```python
from build123d import *

# Parameters (mm, degrees)
EXTRUDE_1_DEPTH     = 4.95
SKETCH_2_R          = 0.5
CUT_EXTRUDE_1_DEPTH = 0.5
CUT_EXTRUDE_2_REACH = 16.197
CUT_EXTRUDE_3_REACH = 16.197
SKETCH_5_R          = 2.8
SKETCH_5_R_2        = 0.4
EXTRUDE_2_DEPTH     = 1.42
CHAMFER_1_SIZE      = 0.5
CHAMFER_1_SIZE2     = 0.466257543


with BuildPart() as part:
    # Эскиз1 → Бобышка-Вытянуть1 (new, symmetric)
    with BuildSketch(Plane(origin=(0, 0, 0), x_dir=(0, 0, -1), z_dir=(1, 0, 0))):
        Polygon((0, 1.59), (-4.55, 1.59), (-4.55, 0.59), (-4.55, 0.34), (-4.55, -1.59), (0, -1.59), align=None)
        Polygon((4.55, 1.59), (0, 1.59), (0, -1.59), (4.55, -1.59), (4.55, 0.34), (4.55, 0.59), align=None)
        Polygon((-4.55, 0.34), (-4.55, 0.59), (-6.25, 0.59), (-6.25, -4.56), (-6, -4.56), (-6, 0.34), align=None)
        Polygon((6.25, 0.59), (4.55, 0.59), (4.55, 0.34), (6, 0.34), (6, -4.56), (6.25, -4.56), align=None)
    extrude(amount=EXTRUDE_1_DEPTH, both=True)

    # Эскиз2 → Вырез-Вытянуть1 (cut)
    with BuildSketch(Plane(origin=(0, 1.59, 0), x_dir=(1, 0, 0), z_dir=(0, 1, 0))):
        with Locations(Location((-4, -3.55, 0), (0, 0, 270))):
            Circle(SKETCH_2_R)
    extrude(amount=-CUT_EXTRUDE_1_DEPTH, mode=Mode.SUBTRACT)

    # Вырез-Вытянуть2: up to this face of the body (flat: up to its plane)
    cut_extrude_2_end = Plane(part.part.faces().sort_by_distance((0, -0.625, 4.55))[0])
    # Эскиз3 → Вырез-Вытянуть2 (cut, up to the picked face)
    with BuildSketch(Plane.XY.offset(6.25), mode=Mode.PRIVATE) as cut_extrude_2_sk1:
        Polygon((-3, -1.59), (-3, 0.59), (-4.95, 0.59), (-4.95, -4.56), (-2.73, -4.56), (-2.73, -1.59), align=None)
    cut_extrude_2_tool1 = split(extrude(cut_extrude_2_sk1.sketch, amount=-CUT_EXTRUDE_2_REACH, mode=Mode.PRIVATE), bisect_by=cut_extrude_2_end, keep=Keep.BOTH, mode=Mode.PRIVATE)
    # Эскиз3 → Вырез-Вытянуть2 (cut, up to the picked face)
    with BuildSketch(Plane.XY.offset(6.25), mode=Mode.PRIVATE) as cut_extrude_2_sk2:
        Polygon((-1, 0.59), (-2, 0.59), (-2, -1.59), (-2.27, -1.59), (-2.27, -4.56), (-0.73, -4.56), (-0.73, -1.59), (-1, -1.59), align=None)
    cut_extrude_2_tool2 = split(extrude(cut_extrude_2_sk2.sketch, amount=-CUT_EXTRUDE_2_REACH, mode=Mode.PRIVATE), bisect_by=cut_extrude_2_end, keep=Keep.BOTH, mode=Mode.PRIVATE)
    # Эскиз3 → Вырез-Вытянуть2 (cut, up to the picked face)
    with BuildSketch(Plane.XY.offset(6.25), mode=Mode.PRIVATE) as cut_extrude_2_sk3:
        Polygon((1, 0.59), (0, 0.59), (0, -1.59), (-0.27, -1.59), (-0.27, -4.56), (1.27, -4.56), (1.27, -1.59), (1, -1.59), align=None)
    cut_extrude_2_tool3 = split(extrude(cut_extrude_2_sk3.sketch, amount=-CUT_EXTRUDE_2_REACH, mode=Mode.PRIVATE), bisect_by=cut_extrude_2_end, keep=Keep.BOTH, mode=Mode.PRIVATE)
    # Эскиз3 → Вырез-Вытянуть2 (cut, up to the picked face)
    with BuildSketch(Plane.XY.offset(6.25), mode=Mode.PRIVATE) as cut_extrude_2_sk4:
        Polygon((3, 0.59), (2, 0.59), (2, -1.59), (1.73, -1.59), (1.73, -4.56), (3.27, -4.56), (3.27, -1.59), (3, -1.59), align=None)
    cut_extrude_2_tool4 = split(extrude(cut_extrude_2_sk4.sketch, amount=-CUT_EXTRUDE_2_REACH, mode=Mode.PRIVATE), bisect_by=cut_extrude_2_end, keep=Keep.BOTH, mode=Mode.PRIVATE)
    # Эскиз3 → Вырез-Вытянуть2 (cut, up to the picked face)
    with BuildSketch(Plane.XY.offset(6.25), mode=Mode.PRIVATE) as cut_extrude_2_sk5:
        Polygon((4.95, 0.59), (4, 0.59), (4, -1.59), (3.73, -1.59), (3.73, -4.56), (4.95, -4.56), align=None)
    cut_extrude_2_tool5 = split(extrude(cut_extrude_2_sk5.sketch, amount=-CUT_EXTRUDE_2_REACH, mode=Mode.PRIVATE), bisect_by=cut_extrude_2_end, keep=Keep.BOTH, mode=Mode.PRIVATE)
    add(cut_extrude_2_tool1.solids().sort_by(Axis((-3.89292, -2.065601, 6.25), (0, 0, -1)))[0], mode=Mode.SUBTRACT)
    add(cut_extrude_2_tool2.solids().sort_by(Axis((-1.5, -2.243838, 6.25), (0, 0, -1)))[0], mode=Mode.SUBTRACT)
    add(cut_extrude_2_tool3.solids().sort_by(Axis((0.5, -2.243838, 6.25), (0, 0, -1)))[0], mode=Mode.SUBTRACT)
    add(cut_extrude_2_tool4.solids().sort_by(Axis((2.5, -2.243838, 6.25), (0, 0, -1)))[0], mode=Mode.SUBTRACT)
    add(cut_extrude_2_tool5.solids().sort_by(Axis((4.389098, -2.138497, 6.25), (0, 0, -1)))[0], mode=Mode.SUBTRACT)

    # Вырез-Вытянуть3: up to this face of the body (flat: up to its plane)
    cut_extrude_3_end = Plane(part.part.faces().sort_by_distance((0, -0.625, -4.55))[0])
    # Эскиз4 → Вырез-Вытянуть3 (cut, up to the picked face)
    with BuildSketch(Plane(origin=(0, 0, -6.25), x_dir=(-1, 0, 0), z_dir=(0, 0, -1)), mode=Mode.PRIVATE) as cut_extrude_3_sk1:
        Polygon((-3, -1.59), (-3, 0.59), (-4.95, 0.59), (-4.95, -4.56), (-2.73, -4.56), (-2.73, -1.59), align=None)
    cut_extrude_3_tool1 = split(extrude(cut_extrude_3_sk1.sketch, amount=-CUT_EXTRUDE_3_REACH, mode=Mode.PRIVATE), bisect_by=cut_extrude_3_end, keep=Keep.BOTH, mode=Mode.PRIVATE)
    # Эскиз4 → Вырез-Вытянуть3 (cut, up to the picked face)
    with BuildSketch(Plane(origin=(0, 0, -6.25), x_dir=(-1, 0, 0), z_dir=(0, 0, -1)), mode=Mode.PRIVATE) as cut_extrude_3_sk2:
        Polygon((-1, 0.59), (-2, 0.59), (-2, -1.59), (-2.27, -1.59), (-2.27, -4.56), (-0.73, -4.56), (-0.73, -1.59), (-1, -1.59), align=None)
    cut_extrude_3_tool2 = split(extrude(cut_extrude_3_sk2.sketch, amount=-CUT_EXTRUDE_3_REACH, mode=Mode.PRIVATE), bisect_by=cut_extrude_3_end, keep=Keep.BOTH, mode=Mode.PRIVATE)
    # Эскиз4 → Вырез-Вытянуть3 (cut, up to the picked face)
    with BuildSketch(Plane(origin=(0, 0, -6.25), x_dir=(-1, 0, 0), z_dir=(0, 0, -1)), mode=Mode.PRIVATE) as cut_extrude_3_sk3:
        Polygon((1, 0.59), (0, 0.59), (0, -1.59), (-0.27, -1.59), (-0.27, -4.56), (1.27, -4.56), (1.27, -1.59), (1, -1.59), align=None)
    cut_extrude_3_tool3 = split(extrude(cut_extrude_3_sk3.sketch, amount=-CUT_EXTRUDE_3_REACH, mode=Mode.PRIVATE), bisect_by=cut_extrude_3_end, keep=Keep.BOTH, mode=Mode.PRIVATE)
    # Эскиз4 → Вырез-Вытянуть3 (cut, up to the picked face)
    with BuildSketch(Plane(origin=(0, 0, -6.25), x_dir=(-1, 0, 0), z_dir=(0, 0, -1)), mode=Mode.PRIVATE) as cut_extrude_3_sk4:
        Polygon((3, 0.59), (2, 0.59), (2, -1.59), (1.73, -1.59), (1.73, -4.56), (3.27, -4.56), (3.27, -1.59), (3, -1.59), align=None)
    cut_extrude_3_tool4 = split(extrude(cut_extrude_3_sk4.sketch, amount=-CUT_EXTRUDE_3_REACH, mode=Mode.PRIVATE), bisect_by=cut_extrude_3_end, keep=Keep.BOTH, mode=Mode.PRIVATE)
    # Эскиз4 → Вырез-Вытянуть3 (cut, up to the picked face)
    with BuildSketch(Plane(origin=(0, 0, -6.25), x_dir=(-1, 0, 0), z_dir=(0, 0, -1)), mode=Mode.PRIVATE) as cut_extrude_3_sk5:
        Polygon((4.95, 0.59), (4, 0.59), (4, -1.59), (3.73, -1.59), (3.73, -4.56), (4.95, -4.56), align=None)
    cut_extrude_3_tool5 = split(extrude(cut_extrude_3_sk5.sketch, amount=-CUT_EXTRUDE_3_REACH, mode=Mode.PRIVATE), bisect_by=cut_extrude_3_end, keep=Keep.BOTH, mode=Mode.PRIVATE)
    add(cut_extrude_3_tool1.solids().sort_by(Axis((3.89292, -2.065601, -6.25), (0, 0, 1)))[0], mode=Mode.SUBTRACT)
    add(cut_extrude_3_tool2.solids().sort_by(Axis((1.5, -2.243838, -6.25), (0, 0, 1)))[0], mode=Mode.SUBTRACT)
    add(cut_extrude_3_tool3.solids().sort_by(Axis((-0.5, -2.243838, -6.25), (0, 0, 1)))[0], mode=Mode.SUBTRACT)
    add(cut_extrude_3_tool4.solids().sort_by(Axis((-2.5, -2.243838, -6.25), (0, 0, 1)))[0], mode=Mode.SUBTRACT)
    add(cut_extrude_3_tool5.solids().sort_by(Axis((-4.389098, -2.138497, -6.25), (0, 0, 1)))[0], mode=Mode.SUBTRACT)

    # Эскиз5 → Бобышка-Вытянуть2 (add)
    with BuildSketch(Plane.XZ.offset(1.59)):
        with Locations(Location((-0.5, 0, 0), (0, 0, 90))):
            Circle(SKETCH_5_R)
        with Locations(Location((-0.5, 0, 0), (0, 0, 270))):
            Circle(SKETCH_5_R_2, mode=Mode.SUBTRACT)
    extrude(amount=EXTRUDE_2_DEPTH)

    # Фаска1
    chamfer_1_edges = [part.edges().sort_by_distance(p)[0] for p in [
        (-0.5, -3.01, -2.8),
    ]]
    chamfer_1_side = [part.faces().sort_by_distance(p)[0] for p in [
        (-0.5, -2.3, -2.8),
    ]]
    chamfer(chamfer_1_edges, length=CHAMFER_1_SIZE, length2=CHAMFER_1_SIZE2, reference=chamfer_1_side[0])


solid = part.part
```
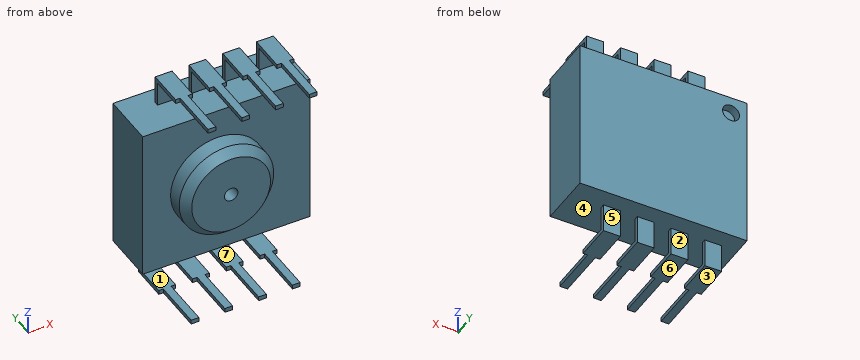
Input: part model. Units: mm. Frame: model coordinates. Face numbers are marked on the shaded views. A direction names the side the tool comes from. Round coordinates to 2 decimals unless told otherwise and drop trailing zeros. Loops run counter-clockwise (first coordinate to the right, second up) from the corner with the lowest first, then second, coordinate; pieces in that order, holes last. Notation, with made-up numbers: M 44,28 L 61,28 A14 ccw 61,45 Z; hole C -39.75,-8 d1. An arc over 180 degrees is marked long. Answer in a Markdown table with one row per item. Add a question column.
1. Mould query, pull axis Z, two halves, no side actions, for the marked faces 1, 2, 3 and 4. Classes: released by +Z, released by -Z, zero draft, split by the parting line, or undercut.
2. Ray query, probe 1 along X at (y, z) = (-2.3, 0); probe 2 along X at (y, z) = (1.35, 3.55); probe 3 along Y at (x, z) = (3.5, -0.5). Return the intervals inside material, ascending.
3. Section A-A (y = -2). Give the number of separate pieces and of enclosed holes in the cut face, and give its area (3 significant figures).
4. Section B-B (z = -4.75). Output: boundary loops of the cut face in (x, y).
5. Section C-C (x = -0.5). Output: boundary loops of the cut face in (y, z).
6. Contact query for flat-ended pins moving along their axis: pin 1 (0.5 mm diameter, centred on x = -3.5, z = -5.5, fed in from -Y); pin 2 (0.8 mm diameter, centred on x = 2.5, z = -6, fed in from +Y); pin 3 (3 mm diameter, centred on x = 0.5, z = 2, fed in from -Y). Output: stop coordinate, or through.
7. Set-up query: the marked faces 5, 6 and 7. Return all of +Z, -Z, +X, -X, +Y, -Y with unobstructed straight access to the full face (end or side cutting, diameter ignored); none if empty.
8. Section D-D (z = 0). Output: boundary loops of the cut face in (x, y).
Values follow:
| question | item | result |
|---|---|---|
| 1 | face 1 | undercut |
| 1 | face 2 | zero draft |
| 1 | face 3 | released by -Z |
| 1 | face 4 | undercut |
| 2 | probe 1 | -3.3 to -0.9, -0.1 to 2.3 |
| 2 | probe 2 | -4.95 to -4.5, -3.5 to 4.95 |
| 2 | probe 3 | -1.59 to 1.59 |
| 3 | separate pieces | 9 |
| 3 | enclosed holes | 1 |
| 3 | area | 25.0 mm^2 |
| 4 | outline | M -4,0.34 L -3,0.34 L -3,0.59 L -4,0.59 Z; M -2,0.34 L -1,0.34 L -1,0.59 L -2,0.59 Z; M 0,0.34 L 1,0.34 L 1,0.59 L 0,0.59 Z; M 2,0.34 L 3,0.34 L 3,0.59 L 2,0.59 Z |
| 5 | outline | M -4.56,6 L 0.34,6 L 0.34,4.55 L -1.59,4.55 L -1.59,2.8 L -2.51,2.8 L -3.01,2.33 L -3.01,0.4 L -1.59,0.4 L -1.59,-0.4 L -3.01,-0.4 L -3.01,-2.33 L -2.51,-2.8 L -1.59,-2.8 L -1.59,-4.55 L 1.59,-4.55 L 1.59,4.55 L 0.59,4.55 L 0.59,6.25 L -4.56,6.25 Z |
| 6 | pin 1 | y = 0.34 |
| 6 | pin 2 | y = 0.59 |
| 6 | pin 3 | y = -3.01 |
| 7 | face 5 | -Z, +X, -X, +Y |
| 7 | face 6 | -Z, +X, -X, +Y, -Y |
| 7 | face 7 | +X, -X, -Y |
| 8 | outline | M -4.95,-1.59 L -3.3,-1.59 L -3.3,-2.51 L -2.83,-3.01 L -0.9,-3.01 L -0.9,-1.59 L -0.1,-1.59 L -0.1,-3.01 L 1.83,-3.01 L 2.3,-2.51 L 2.3,-1.59 L 4.95,-1.59 L 4.95,1.59 L -4.95,1.59 Z |
